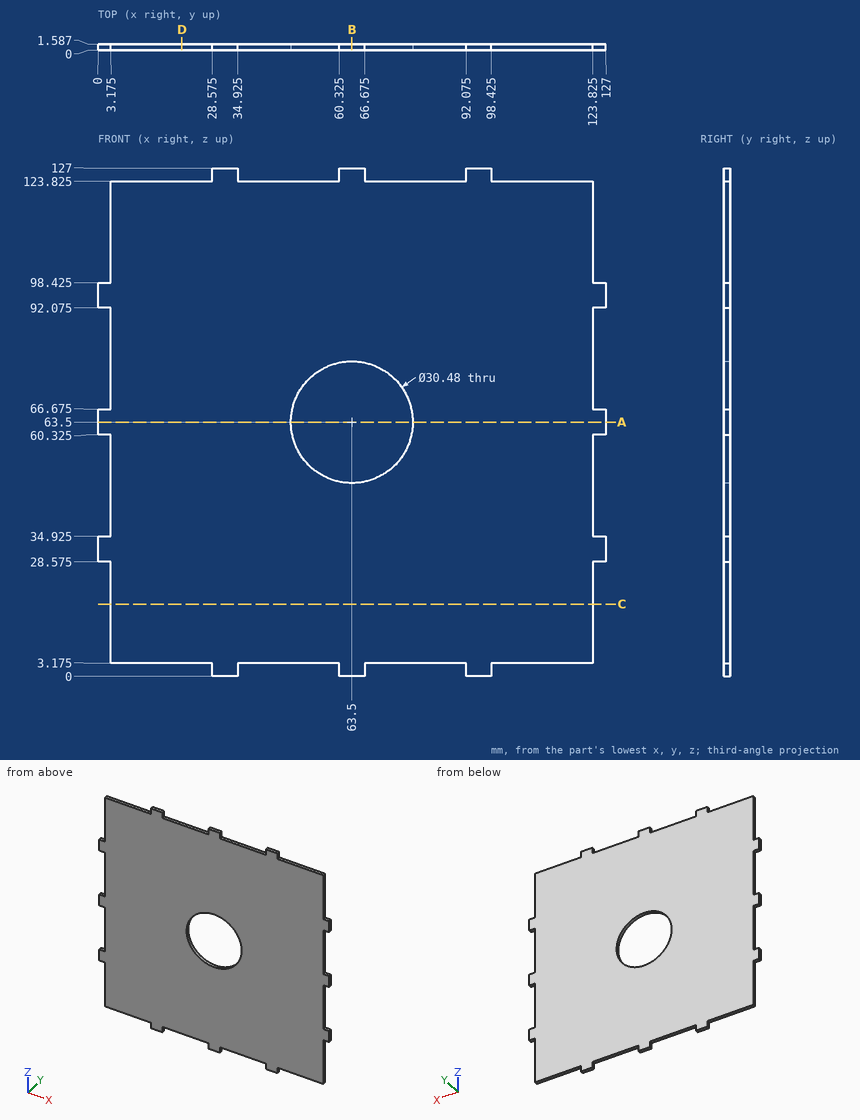
Can you work these out from the drawing? Everything is in mm from the part's minimum corner. Round coordinates to 2 decimals unless told otherwise and drop trailing zeros. Order: outer loops, then holes, each group sorted by start corner. A loop starts at its lowest first (then second) coordinate and runs counter-clockwise, first axis right, second up. Notation, with made-up numbers: M 71.25,14 L 83.25,14 A18 cw 83.25,26 Z; hole C 87.25,-11.75 d8. An arc over 180 degrees is marked long. One line per question, with ' | ' between items.
1) I need wall thicknesses on line 1 along X through (y, z) = (0.95, 63.5); line 2 along X through (y, z) = (0.8, 38.5) (1 decimal). Which ranges of each line are inside material? Lowest first, please.
Working result:
line 1: 0 to 48.26, 78.74 to 127 | line 2: 3.2 to 123.8
2) I want a section at D-D, the plane x = 21. Write out the boundary of the cut face in (y, z) (1 decimal).
Working result:
outline: M 0,3.2 L 1.6,3.2 L 1.6,123.8 L 0,123.8 Z
3) I want a section at A-A, the plane z = 63.5. Write out the boundary of the cut face in (x, y).
Working result:
outline: M 0,0 L 48.26,0 L 48.26,1.59 L 0,1.59 Z; M 78.74,0 L 127,0 L 127,1.59 L 78.74,1.59 Z
4) I want a section at C-C, the plane z = 18. Write out the boundary of the cut face in (x, y) (1 decimal).
Working result:
outline: M 3.2,0 L 123.8,0 L 123.8,1.6 L 3.2,1.6 Z
5) I want a section at B-B, the plane x = 63.5. Write out the boundary of the cut face in (y, z).
Working result:
outline: M 0,0 L 1.59,0 L 1.59,48.26 L 0,48.26 Z; M 0,78.74 L 1.59,78.74 L 1.59,127 L 0,127 Z
6) For pin 1 Ø0.8 at (x, y) = (11, 1) entering from -Z (1 decimal); pin 2 Ø0.5 at (y, z) = (0.5, 125.5) entering from -X (1 decimal); pin 3 Ø0.5 at (y, z) = (0.5, 12.5) entering from -X (1 decimal), each with a flat end and sliding along its axis, tell me the tip position at first contact or that it passes through.
Working result:
pin 1: z = 3.2 | pin 2: x = 28.6 | pin 3: x = 3.2
